Check sheet for the modelled part. Datum: model origin and axes. Units: mm. A direction names the side the tool comes from. Coordinates: 2 decimals unless noted, no trailing zeros. Loops run counter-clockwise (first coordinate to the right, second up) from the corner with the lowest first, then second, coordinate; pieces in that order, holes last. Notation, with made-up numbers: (-7.75, -37.75) - (23.25, -37.75) arc R15 cw to (23.25, -8.75) - close; hole circle Ø9 at (-20, 19). An arc over 180 degrees is marked (long way). Answer as a JSON object with one key per item and string values. Group by question number.
from build123d import *

# Parameters (mm, degrees)
F0_R     = 5.4
F1_DEPTH = 1.5
F3_DEPTH = 1.5
F4_DEPTH = 1.5
F6_DEPTH = 1.5
F7_DEPTH = 1.5
F8_R     = 1


with BuildPart() as f1:
    # F0 (on Top) → F1 (new body, symmetric)
    with BuildSketch(Plane.XY):
        Circle(F0_R)
        with BuildLine():
            ThreePointArc((1.525, 2.1057955741), (2.3157072354, 1.1821590418), (2.6, 0))
            ThreePointArc((2.6, 0), (2.3157072354, -1.1821590418), (1.525, -2.1057955741))
            ThreePointArc((1.525, -2.1057955741), (0, -2.6), (-1.525, -2.1057955741))
            ThreePointArc((-1.525, -2.1057955741), (-2.6, 0), (-1.525, 2.1057955741))
            ThreePointArc((-1.525, 2.1057955741), (0, 2.6), (1.525, 2.1057955741))
        make_face(mode=Mode.SUBTRACT)
        with BuildLine():
            ThreePointArc((1.525, -2.1057955741), (2.3157072354, -1.1821590418), (2.6, 0))
            ThreePointArc((2.6, 0), (2.3157072354, 1.1821590418), (1.525, 2.1057955741))
            Line((1.525, 2.1057955741), (1.525, -2.1057955741))
        make_face()
        with BuildLine():
            Line((-1.525, -2.1057955741), (-1.525, 2.1057955741))
            ThreePointArc((-1.525, 2.1057955741), (-2.6, 0), (-1.525, -2.1057955741))
        make_face()
    extrude(amount=F1_DEPTH, both=True)

    # F2 (on Top) → F3 (join, through all)
    with BuildSketch(Plane.XY):
        Polygon((-2, 4.724830389), (0, 4.724830389), (2, 4.724830389), (3.0572322193, 35), (0, 35), (-3.0572322193, 35), align=None)
    extrude(amount=F3_DEPTH)

    # F4 (add, through all): a face of the model
    f4_faces = [f1.faces().sort_by_distance(p)[0] for p in [
        (0, 21.149058398, 0),
    ]]
    extrude(f4_faces, amount=F4_DEPTH)

    # F5 (on Top) → F6 (join, through all)
    with BuildSketch(Plane.XY):
        Polygon((0, 47.5), (-7.5, 35), (7.5, 35), align=None)
    extrude(amount=F6_DEPTH)

    # F7 (add, through all): a face of the model
    f7_faces = [f1.faces().sort_by_distance(p)[0] for p in [
        (0, 39.1666666667, 0),
    ]]
    extrude(f7_faces, amount=F7_DEPTH)

    # F8
    f8_edges = [f1.edges().sort_by_distance(p)[0] for p in [
        (0, 47.5, 0),
        (-7.5, 35, 0),
        (7.5, 35, 0),
    ]]
    fillet(f8_edges, radius=F8_R)


solid = f1.part
1. Sectioned sample at D-D on y = 9.5. Record the cut outline in (x, z).
2. Gauge pin test, flat ends, axial feed: pin 1 (1.5 mm diameter, centred on x = 5, z = -0.5, fed in from -Y); pin 2 (6 mm diameter, centred on x = -3.5, y = 27, fed in from -Z). Record the tip position at first contact, or that the pin passes through.
3. Sectioned sample at C-C on y = 0. Record the cut outline in (x, z) (3 decimals), plus the area to 4 significant figures.
4. Sectioned sample at B-B on z = 0.1. Record the cut outline in (x, y) (1 decimal), plus the area to 3 significant figures.
5. Sectioned sample at A-A on x = 0. Record the cut outline in (y, z).
6. Material ranges on line 1 (Y direction, x = -4, z = -0.8); line 2 (Y direction, x = 4.5, z = 0.05); line 3 (X direction, y = 2, z = 0.25) (3 decimals), recorded low to high.
7. Access from +Z, -Z, +X, -X, +Y, -Y to the whole of each face (thin tool, end or side, straight path). Record for faces 1 (the face through (-1.525, 0, 0)), 2 (the face through (-3.684, 41.36, 0.021)), 3 (the face through (4, 35, 0)), 4 (the face through (0, 21, -1.5)), 5 (the face through (-4, 35, 0)).
Answers follow:
{
 "1": {"outline": "(-2.17, -1.5) - (2.17, -1.5) - (2.17, 1.5) - (-2.17, 1.5) - close"},
 "2": {"pin 1": "stops at y = -3.33", "pin 2": "stops at z = -1.5"},
 "3": {"outline": "(-5.4, -1.5) - (-1.525, -1.5) - (-1.525, 1.5) - (-5.4, 1.5) - close; (1.525, -1.5) - (5.4, -1.5) - (5.4, 1.5) - (1.525, 1.5) - close", "area": "23.25 mm^2"},
 "4": {"outline": "(-6.6, 36.5) arc R1 ccw to (-5.7, 35) - (-3.1, 35) - (-2, 5) arc R5.4 ccw (long way) to (2, 5) - (3.1, 35) - (5.7, 35) arc R1 ccw to (6.6, 36.5) - (0.9, 46.1) arc R1 ccw to (-0.9, 46.1) - close; hole (-1.5, -2.1) arc R2.6 ccw to (1.5, -2.1) - (1.5, 2.1) arc R2.6 ccw to (-1.5, 2.1) - close", "area": "319 mm^2"},
 "5": {"outline": "(-5.4, -1.5) - (-2.6, -1.5) - (-2.6, 1.5) - (-5.4, 1.5) - close; (2.6, -1.5) - (46.56, -1.5) - (46.56, 1.5) - (2.6, 1.5) - close"},
 "6": {"line 1": "y = -3.63 to 3.63, 35 to 40.83", "line 2": "y = -2.98 to 2.98, 35 to 40", "line 3": "x = -5.016 to -1.525, 1.525 to 5.016"},
 "7": {"face 1": "+Z, -Z", "face 2": "+Z, -Z, -X, +Y", "face 3": "+Z, -Z, +X", "face 4": "-Z, +X, -X, +Y, -Y", "face 5": "+Z, -Z, -X"}
}
